Geometry: final body of the model. Coordinates: model frame, mm. Face numbers are marked on the shaded views. A direction names the side the tool comes from. Give positions to 0.01 mm unless a question says otherwise; leave off trailing zeros. Write each loop counter-clockwise with the first axis right and the second up, starting at its lowest first coordinate (ties: lowest second). Pieces come first, ordered by that corner, then holes. Notation, with made-up numbers: (-35.75, 67) -> (-7.75, 67) arc R29 ccw to (-7.75, 93) -> close; hole circle Ø4 at (18, 81). An arc over 180 degrees is marked (long way). Answer as a JSON object with one key per item and string values.
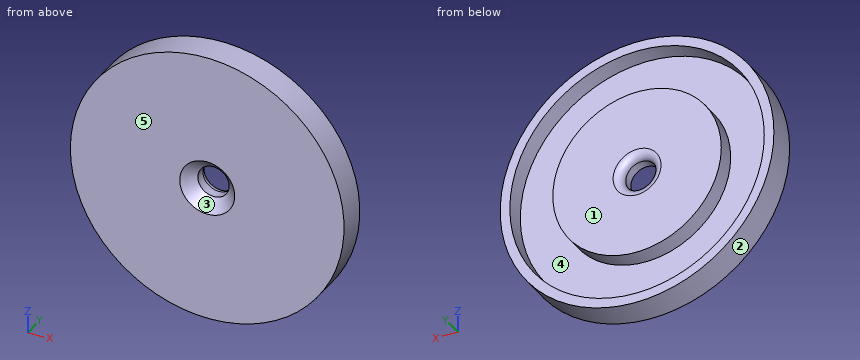
Autodesk Inventor part; units mm, degrees
ref_plane "YZ Plane" through (0, 0, 0) normal (1, 0, 0) x (0, 1, 0)
ref_plane "XZ Plane" through (0, 0, 0) normal (0, 1, 0) x (-1, 0, 0)
ref_plane "XY Plane" through (0, 0, 0) normal (0, 0, 1) x (1, 0, 0)
sketch "Sketch1" plane through (0, 0, 0) normal (0, 1, 0) x (-1, 0, 0)
  circle A0 centre (0, 0) radius 21.35
  circle A1 centre (0, 0) radius 14.25
  circle A2 centre (0, 0) radius 23.15
  dimension "d0" = 42.7
  dimension "d1" = 28.5
  dimension "d3" = 1.8
extrude "Extrusion1" add sketch "Sketch1" along normal blind 5
extrude "Extrusion2" add sketch "Sketch1" along normal blind 2 contours A0
draft "FaceDraft1" angle 3.3 pull direction (0, 1, 0) faces at (-21.0735, 4, -3.4248) fixed edges at (21.35, 2, 0)
hole "Hole1" at (0, 0, 0) direction (0, 1, 0) diameter 5.3 end through all
chamfer "Chamfer1" distance 2 angle 45 1 edges at (0, 0, 2.65)
fillet "Fillet1" radius 1.4 1 edges at (0, 5, 2.65)
properties part number "Cap V2 (App V5)"
Q1. Cut plane A-A (x = 0). Return the cut outline in (y, z).
Values:
{"outline": "(0, -23.15) -> (5, -23.15) -> (5, -21.52) -> (2, -21.35) -> (2, -14.25) -> (5, -14.25) -> (5, -4.05) arc R1.4 ccw to (3.6, -2.65) -> (2, -2.65) -> (0, -4.65) -> close; (0, 4.65) -> (2, 2.65) -> (3.6, 2.65) arc R1.4 ccw to (5, 4.05) -> (5, 14.25) -> (2, 14.25) -> (2, 21.35) -> (5, 21.52) -> (5, 23.15) -> (0, 23.15) -> close"}
Q2. Cut plane B-B (z = 0). Return the cut outline in (x, y), and give its area (3 significant figures).
Values:
{"outline": "(-23.15, 0) -> (-4.65, 0) -> (-2.65, 2) -> (-2.65, 3.6) arc R1.4 ccw to (-4.05, 5) -> (-14.25, 5) -> (-14.25, 2) -> (-21.35, 2) -> (-21.52, 5) -> (-23.15, 5) -> close; (2.65, 2) -> (4.65, 0) -> (23.15, 0) -> (23.15, 5) -> (21.52, 5) -> (21.35, 2) -> (14.25, 2) -> (14.25, 5) -> (4.05, 5) arc R1.4 ccw to (2.65, 3.6) -> close", "area": "157 mm²"}
Q3. Set-up query: the marked faces 4 and 5. Return all of +Z, -Z, +X, -X, +Y, -Y with unobstructed straight access to the full face (end or side cutting, diameter ignored); none if empty.
Values:
{"face 4": "+Y", "face 5": "+Z, -Z, +X, -X, -Y"}
Q4. First-contact query: P1, Ø5, axis at x = 17, z = 11.5, coming from the -Y side; P2, Ø1, axis at x = 3.5, y = 1, coming from the +Z side; P3, Ø2, axis at x = -12.5, y = 0.5, coming from the +Z side; P4, Ø1.5, axis at x = -5.5, y = 1, coming from the -Z side. Flat tips, straight axial feed; report the tip coordinate or a pass-through.
Values:
{"P1": "y = 0", "P2": "z = 22.95", "P3": "z = 20.09", "P4": "z = -22.66"}
Q5. Mould query, pull axis X, two halves, no side actions, for the marked faces 1, 2 and 3. Classes: pulls with the +X half, pulls with the -X half, needs draft (parallel to the pull), parting line crosses it, or undercut.
Values:
{"face 1": "needs draft", "face 2": "parting line crosses it", "face 3": "undercut"}
Q6. Material intervals for L1, parallel to X at y = 2.2, z = 10; L2, parallel to Y at x = -14, z = 5; L3, parallel to X at y = 3.2, z = -3, sorted ascending. Write a range as from..to.
Values:
{"L1": "-20.88..-18.88, -10.15..10.15, 18.88..20.88", "L2": "0..2", "L3": "-22.95..-21.21, -13.93..13.93, 21.21..22.95"}
Q7. Cut plane C-C (y = 2.55). Return the cut outline in (x, z), and give its area (3 significant figures).
Values:
{"outline": "circle Ø46.3 at (0, 0); circle Ø28.5 at (0, 0); hole circle Ø42.76 at (0, 0); hole circle Ø5.3 at (0, 0)", "area": "863 mm²"}
